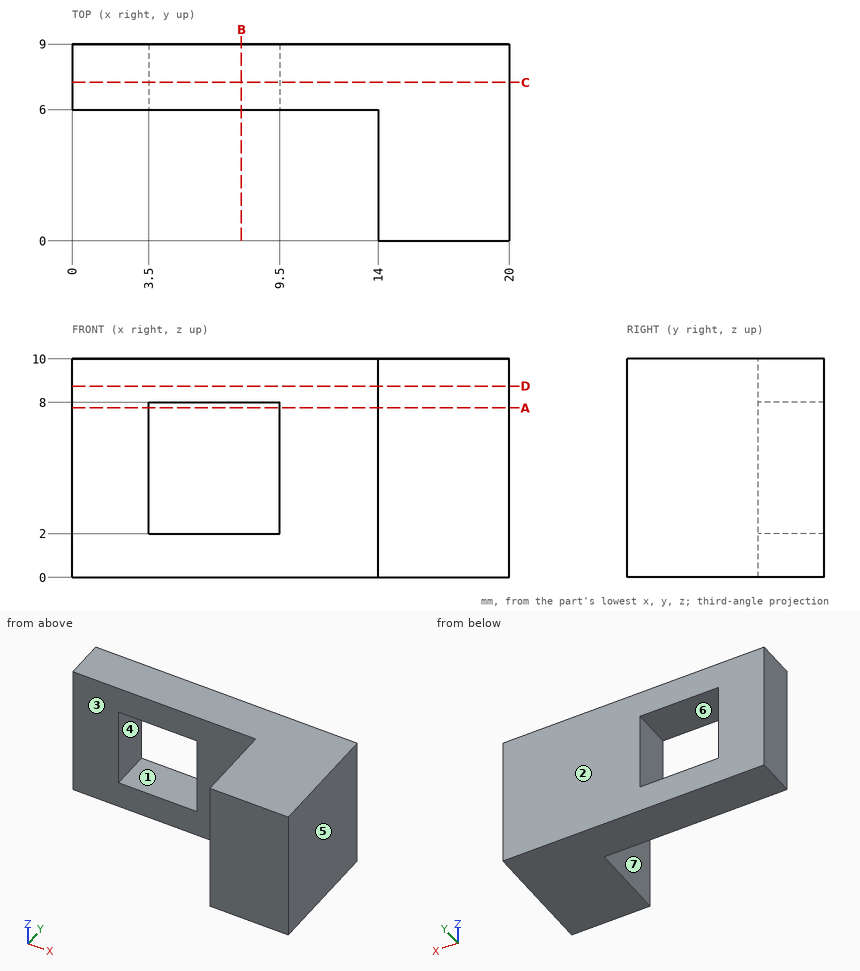
The drawing under review shows one solid part. Ordinate dimensions are in mm from its lowest x, y, z. A direction names the side the tool comes from. Round coordinates to 2 decimals unless told otherwise and drop trailing zeros. Loops run counter-clockwise (first coordinate to the right, second up) from the corner with the lowest first, then second, coordinate; pieces in that order, holes last. Notation, with made-up numbers: M 50,19 L 65,19 A33 ccw 65,52 Z; hole C 4.25,12.5 d3. An arc over 180 degrees is marked long. Answer as CSV lines item,"result". Start each with the question number.
Item 1: For the marked faces 1, 2 and 3, list the 3-axis set-ups (+Z, -Z, +X, -X, +Y, -Y) from which the entire face can be reached by the end or side of a thin tool; tool diameter is ignored.
Item 2: Insertion check: P1, Ø1, axis at x = 3.5, z = 2.5, coming from the -Y side; P2, Ø1.5, axis at y = 3, z = 4, coming from the -X side. Each pin has a flat end and moves straight along its axis. Give the tip position at first contact, or say it passes through.
Item 3: Wall thickness on line 1 (X direction, y = 7.5, z = 3); line 2 (Z direction, x = 6.25, y = 7); line 3 (Y direction, x = 12.5, z = 8.5): over which ranges is each line inside the solid? List them lowest first. Write a range as [from, to].
Item 4: Mouldability with a two-part tool opening along X and no side actions: class the marked faces 4, 5, 6 and 7 as released by +X, released by -X, zero draft, split by the parting line, or undercut.
Item 5: Consider section C-C (y = 7.25). Write out the cut boundary in (x, z).
Item 6: Consider section B-B (x = 7.75). Write out the cut boundary in (y, z), then the cut area to 3 significant figures.
Item 7: Consider section A-A (z = 7.75). Write out the cut boundary in (x, y).
Item 8: Consider section D-D (z = 8.75). Write out the cut boundary in (x, y).
Answer:
1,face 1,"+Y, -Y"
1,face 2,"+Z, -Z, +X, -X, +Y"
1,face 3,"+Z, -Z, -X, -Y"
2,P1,"stops at y = 6"
2,P2,"stops at x = 14"
3,line 1,"x = [0, 3.5], [9.5, 20]"
3,line 2,"z = [0, 2], [8, 10]"
3,line 3,"y = [6, 9]"
4,face 4,"undercut"
4,face 5,"released by +X"
4,face 6,"undercut"
4,face 7,"released by -X"
5,outline,"M 0,0 L 20,0 L 20,10 L 0,10 Z; hole M 3.5,2 L 9.5,2 L 9.5,8 L 3.5,8 Z"
6,outline,"M 6,0 L 9,0 L 9,2 L 6,2 Z; M 6,8 L 9,8 L 9,10 L 6,10 Z"
6,area,"12.0 mm^2"
7,outline,"M 0,6 L 3.5,6 L 3.5,9 L 0,9 Z; M 9.5,6 L 14,6 L 14,0 L 20,0 L 20,9 L 9.5,9 Z"
8,outline,"M 0,6 L 14,6 L 14,0 L 20,0 L 20,9 L 0,9 Z"
